```python
from build123d import *

# Parameters (mm, degrees)
CYLINDER034_R     = 3
CYLINDER034_DEPTH = 3
BOX013_W          = 9.525
BOX013_H          = 9.525
BOX013_DEPTH      = 3


with BuildPart() as cylinder034:
    # Cylinder034 → Cylinder034 (new body)
    with BuildSketch(Plane(origin=(6.35, 6.35, 0), x_dir=(1, 0, 0), z_dir=(0, 0, 1))):
        Circle(CYLINDER034_R)
    extrude(amount=CYLINDER034_DEPTH)


with BuildPart() as m6_nut:
    # Box013 → Box013 (new body)
    with BuildSketch(Plane(origin=(1.62052, 1.55448, 0), x_dir=(1, 0, 0), z_dir=(0, 0, 1))):
        with Locations((4.7625, 4.7625)):
            Rectangle(BOX013_W, BOX013_H)
    extrude(amount=BOX013_DEPTH)

    # Cut011: cut Cylinder034
    add(cylinder034.part, mode=Mode.SUBTRACT)


with BuildPart() as m6_nut_1:
    # Cut011 placement: moved
    add(m6_nut.part.moved(Location((0, -40.41648, 0))))


solid = m6_nut_1.part
```
Input: part model. Units: mm. Frame: model coordinates. Give positions to 0.01 mm unless a question says otherwise; leave off trailing zeros. Write each loop counter-clockwise with the first axis right and the second up, starting at its lowest first coordinate (ties: lowest second). Pieces come first, ordered by that corner, then holes. Notation, with made-up numbers: (21.5, 77) - (55.5, 77) arc R21 ccw to (55.5, 89) - close; hole circle Ø7 at (83, 82.5). An arc over 180 degrees is marked (long way). Write item = value, one per line. Start each with the question number.
1. Section query A-A, the plane x = 6.35. Output: boundary loops of the cut face in (y, z), then the cut area to 3 significant figures.
2. Section query C-C, the plane z = 2. Output: boundary loops of the cut face in (x, y), then the cut area to 3 significant figures.
3. Section query B-B, the plane y = -34.5. Output: boundary loops of the cut face in (x, z).
4. Ray query, L1, parallel to Y at x = 6.35, z = 2.3; L2, parallel to X at y = -34, z = 1.2; L3, parallel to X at y = -36.5, z = 0.85. Return the intervals inside material, ascending.
5. Mould query, pull axis X, two halves, no side actions, for faces 1 (the flat face through (1.621, -34, 1)), 2 (the flat face through (6, -29.337, 1)), 3 (the cylindrical face through (5.96, -31.09, 1.48)). Classes: released by +X, released by -X, zero draft, split by the parting line, or undercut.
Check sheet entries:
q1.outline = (-38.86, 0) - (-37.07, 0) - (-37.07, 3) - (-38.86, 3) - close; (-31.07, 0) - (-29.34, 0) - (-29.34, 3) - (-31.07, 3) - close
q1.area = 10.6 mm2
q2.outline = (1.62, -38.86) - (11.15, -38.86) - (11.15, -29.34) - (1.62, -29.34) - close; hole circle Ø6 at (6.35, -34.07)
q2.area = 62.5 mm2
q3.outline = (1.62, 0) - (3.38, 0) - (3.38, 3) - (1.62, 3) - close; (9.32, 0) - (11.15, 0) - (11.15, 3) - (9.32, 3) - close
q4.L1 = -38.86 to -37.07, -31.07 to -29.34
q4.L2 = 1.62 to 3.35, 9.35 to 11.15
q4.L3 = 1.62 to 4.6, 8.1 to 11.15
q5.face_1 = released by -X
q5.face_2 = zero draft
q5.face_3 = undercut
